Build history of the part. All positions in model axes, mm. A direction names the side the tool comes from. Coordinates: 2 decimals unless noted, no trailing zeros. Loops run counter-clockwise (first coordinate to the right, second up) from the corner with the lowest first, then second, coordinate; pieces in that order, holes last.
(1) Two-plate mould, pull along X, no slides. Class faces 3 (the face through (-138, -197, -32.455)), 4 (the face through (-307.037, -193, 234)), 5 (the face through (-142, 0, 234)): pulls with the +X half, pulls with the -X half, needs draft (parallel to the pull), parting line crosses it, or undercut.
(2) Slice it at A-A (x = -45.5). Give the cut face in (y, z), and give its area (3 significant figures).
(3) Slice it at C-C (y = -130). Give the cut face in (x, z).
(4) Slice it at B-B (z = 487.5). Give the cut face in (x, y), and give its area (3 significant figures).
(5) Tool access for faces 1 (the face through (-289.257, -202, 234)), 2 (the face through (27.637, -193, 234)): list every direction of +Z, -Z, +X, -X, +Y, -Y with a clear straight run to the whole face (end or side of a thin tool).
(6) Wall check: L1, parallel to Z at x = -285, y = -154; L2, parallel to X at y = -134, z = 309; L3, parallel to Y at x = -182.5, z = 436. Give the ranges that are in metal, low to high.
(7) Flat gauge pins, fed straight in: P1, Ø4, axis at x = -219, z = 243, coming from the -Y side; P2, Ø5, axis at x = -177.5, z = 64, coming from the +Y side. Where does each tip first touch, or does it go through?
from build123d import *

# Parameters (mm, degrees)
F0_W     = 55.2740842104
F0_H     = 94.0575622953
F1_DEPTH = 381
F2_DEPTH = 279.4
F3_W     = 334.6740842104
F3_H     = 381
F4_DEPTH = 482.6
F5_T     = -17.78


with BuildPart() as f1:
    # F0 (on Front) → F1 (new body)
    with BuildSketch(Plane.XZ):
        with Locations((0, -3.2065075357)):
            Rectangle(F0_W, F0_H)
    extrude(amount=F1_DEPTH)

    # F2 (add): a face of the model
    f2_faces = [f1.faces().sort_by_distance(p)[0] for p in [
        (-27.6370421052, -190.5, -3.2065075357),
    ]]
    extrude(f2_faces, amount=F2_DEPTH)

    # F3 (on face) → F4 (join)
    with BuildSketch(Plane.XY.offset(43.822273612)):
        with Locations((-139.7, -190.5)):
            Rectangle(F3_W, F3_H)
    extrude(amount=F4_DEPTH)

    # F5
    f5_openings = [f1.faces().sort_by_distance(p)[0] for p in [
        (-139.7, -381, 238.093492),
    ]]
    offset(amount=F5_T, openings=f5_openings)


solid = f1.part
Response values:
1. face 3: undercut
1. face 4: pulls with the -X half
1. face 5: needs draft
2. outline: (-381, -50.24) - (0, -50.24) - (0, 526.42) - (-381, 526.42) - (-381, 508.64) - (-17.78, 508.64) - (-17.78, -32.46) - (-381, -32.46) - close
2. area: 23,200 mm2
3. outline: (-307.04, -50.24) - (27.64, -50.24) - (27.64, 526.42) - (-307.04, 526.42) - close; hole (-289.26, -32.46) - (9.86, -32.46) - (9.86, 508.64) - (-289.26, 508.64) - close
4. outline: (-307.04, -381) - (-289.26, -381) - (-289.26, -17.78) - (9.86, -17.78) - (9.86, -381) - (27.64, -381) - (27.64, 0) - (-307.04, 0) - close
4. area: 18,900 mm2
5. face 1: -Y
5. face 2: +Z, -Z, +X, +Y, -Y
6. L1: z = -50.24 to -32.46, 508.64 to 526.42
6. L2: x = -307.04 to -289.26, 9.86 to 27.64
6. L3: y = -17.78 to 0
7. P1: stops at y = -17.78
7. P2: stops at y = 0
